Read the model definition and answer for the solid it produces. Units are mm, in the model's axes. Face numbers are marked on the shaded views. Coordinates: 2 decimals unless noted, no trailing zeros. Write each loop counter-clockwise with the first axis right and the second up, starting at its lowest first coordinate (ties: lowest second). Pieces come first, ordered by that corner, then holes. Notation, with made-up numbers: M 6,2.5 L 33,2.5 A21 ccw 33,30.5 Z; hole C -6,44.25 d2. An arc over 180 degrees is marked long. Write item = value, one per line.
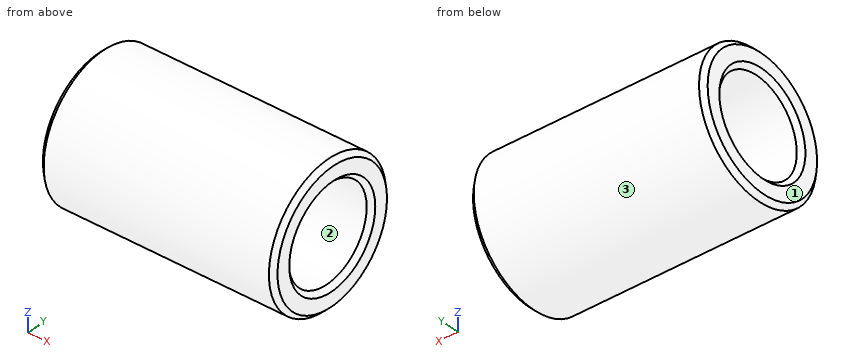
Autodesk Inventor part; units mm, degrees
ref_plane "YZ Plane" through (0, 0, 0) normal (1, 0, 0) x (0, 1, 0)
ref_plane "XZ Plane" through (0, 0, 0) normal (0, 1, 0) x (-1, 0, 0)
ref_plane "XY Plane" through (0, 0, 0) normal (0, 0, 1) x (1, 0, 0)
sketch "_____1" plane through (0, 0, 0) normal (0, 0, 1) x (1, 0, 0)
  line L0 (10, 0) -> (0, 0)
  line L1 (0, 0) -> (0, 2.8)
  line L2 (0, 2.8) -> (0.2, 3)
  line L3 (0.2, 3) -> (9.8, 3)
  line L4 (9.8, 3) -> (10, 2.8)
  line L5 (10, 2.8) -> (10, 0)
  line L6 (10, 0) -> (0, 0)
revolve "Revolution1" add sketch "_____1" angle 360 about axis through (10, 0, 0) along (1, 0, 0)
sketch "_____2" plane through (0, 0, 0) normal (0, 0, 1) x (1, 0, 0)
  line L0 (20, 0) -> (-20, 0)
  line L1 (0, 0) -> (0, 2.2)
  line L2 (0, 2.2) -> (0.2, 2)
  line L3 (0.2, 2) -> (9.8, 2)
  line L4 (9.8, 2) -> (10, 2.2)
  line L5 (10, 2.2) -> (10, 0)
  line L6 (10, 0) -> (0, 0)
revolve "Revolution2" cut sketch "_____2" angle 360 about axis through (20, 0, 0) along (1, 0, 0)
properties part number "C-KNCLA4-6-10"
Item 1: Find section A-A (z = 0). Determine the outline of the cut face in (x, y), and give its area (3 significant figures).
Worked answers:
outline = M 0,-2.8 L 0.2,-3 L 9.8,-3 L 10,-2.8 L 10,-2.2 L 9.8,-2 L 0.2,-2 L 0,-2.2 Z; M 0,2.2 L 0.2,2 L 9.8,2 L 10,2.2 L 10,2.8 L 9.8,3 L 0.2,3 L 0,2.8 Z
area = 19.8 mm²
Item 2: A flat-ended cylindrical pin translates along its axis: pin 1 (1.5 mm diameter, centred on y = 2, z = -2, fed in from +X). Find the tip coordinate at first contact, or state that the pin passes through.
Worked answers:
pin_1 = 10
Item 3: For a pull along Z with two mould halves and no side action, classify the marked faces 1, 2 and 3 as released by +Z, released by -Z, zero draft, split by the parting line, or undercut.
Worked answers:
face_1 = zero draft
face_2 = undercut
face_3 = split by the parting line
Item 4: Find section C-C (x = 2.75). Determine the outline of the cut face in (y, z).
Worked answers:
outline = C 0,0 d6; hole C 0,0 d4
Item 5: Consider line 1 along Z through (x, y) = (3.5, 0); line 2 along Z through (x, y) = (1, 1.1); line 3 along Y through (x, z) = (6.25, -0.7). Determine where each line is inside the solid, lowest interval first. Write a range as from..to.
Worked answers:
line_1 = -3..-2, 2..3
line_2 = -2.79..-1.67, 1.67..2.79
line_3 = -2.92..-1.87, 1.87..2.92
